Answer from the drawing. Dimensions are ordinates in mm from the lowest x, y and z of the part. A direction names the side the tool comes from. Coordinates: 2 decimals unless noted, no trailing zeros. Loops run counter-clockwise (first coordinate to the right, second up) from the corner with the lowest first, then second, coordinate; pieces in that order, holes last. Notation, with made-up numbers: M -19.75,89.5 L 27.25,89.5 A27 ccw 27.25,123.5 Z; hole C 58,73.5 d7. An arc over 180 degrees is marked long. One line per item, written item: value. Start each with the question number.
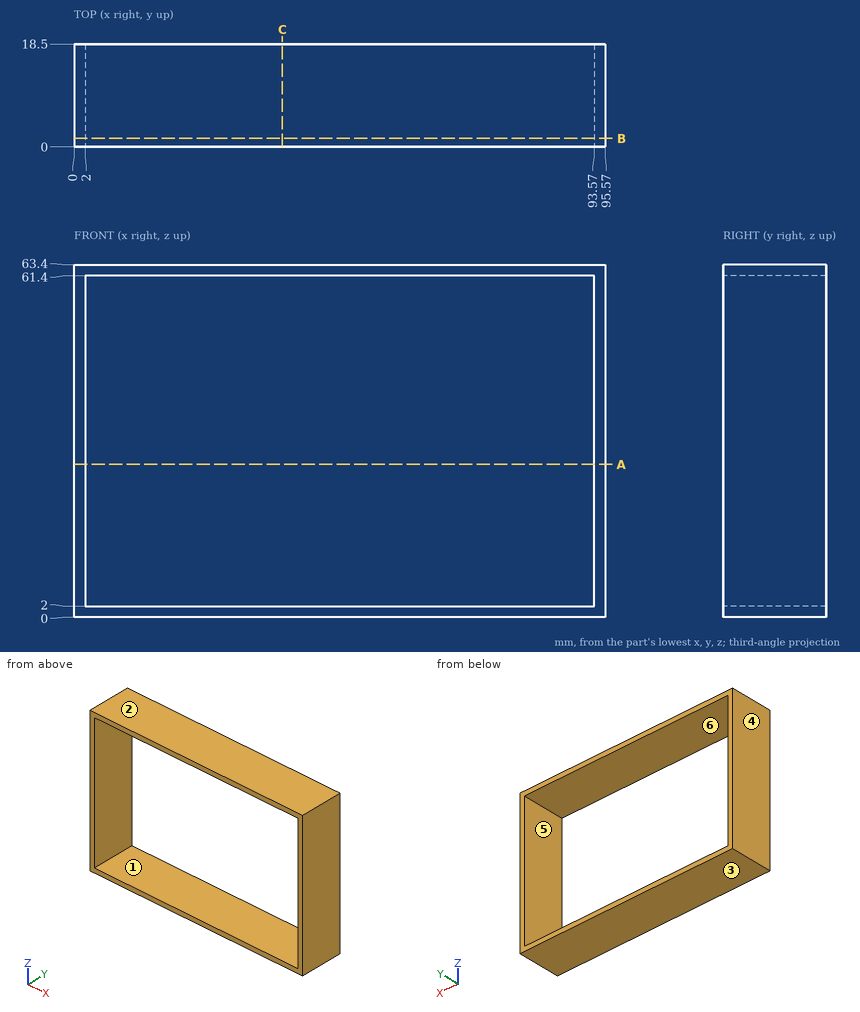
1) Section A-A (z = 27.5) is taken. Determine the outline of the cut face in (x, y), then the cut area to 3 significant figures.
2) A tool of negligible diameter and unlimited length cuts with its end or side. For the marked faces 1 and 2, from which of +Z, -Z, +X, -X, +Y, -Y can it reach the whole face along a straight path? Write none if from no direction.
3) Section B-B (y = 1.5) is taken. Determine the outline of the cut face in (x, z).
4) For a pull along Z with two mould halves and no side action, classify the marked faces 3, 4, 5 and 6 as released by +Z, released by -Z, zero draft, split by the parting line, or undercut.
5) Section C-C (x = 37.5) is taken. Determine the outline of the cut face in (y, z), then the cut area to 3 significant figures.
6) Consider line 1 along Z through (x, y) = (87, 1.25); line 2 along X through (y, z) = (3.5, 53). Determine where each line is inside the solid, lowest interval first.
Results found:
1. outline: M 0,0 L 2,0 L 2,18.5 L 0,18.5 Z; M 93.57,0 L 95.57,0 L 95.57,18.5 L 93.57,18.5 Z
1. area: 74.0 mm²
2. face 1: +Y, -Y
2. face 2: +Z, +X, -X, +Y, -Y
3. outline: M 0,0 L 95.57,0 L 95.57,63.4 L 0,63.4 Z; hole M 2,2 L 93.57,2 L 93.57,61.4 L 2,61.4 Z
4. face 3: released by -Z
4. face 4: zero draft
4. face 5: undercut
4. face 6: undercut
5. outline: M 0,0 L 18.5,0 L 18.5,2 L 0,2 Z; M 0,61.4 L 18.5,61.4 L 18.5,63.4 L 0,63.4 Z
5. area: 74.0 mm²
6. line 1: z = 0 to 2, 61.4 to 63.4
6. line 2: x = 0 to 2, 93.57 to 95.57
